For this review, take the finished solid that the model builds, in its own axes (mm). Coordinates: 2 decimals unless noted, no trailing zeros. Loops run counter-clockwise (first coordinate to the right, second up) from the corner with the lowest first, then second, coordinate; pieces in that order, holes last. Notation, with made-up numbers: (57.5, -33.5) -> (88.5, -33.5) arc R28 cw to (88.5, -5.5) -> close; hole circle Ø10 at (24, -35.5). An arc over 180 degrees is marked (long way). Use a Markdown table: item, result.
Autodesk Inventor part; units mm, degrees
ref_plane "YZ Plane" through (0, 0, 0) normal (1, 0, 0) x (0, 1, 0)
ref_plane "XZ Plane" through (0, 0, 0) normal (0, 1, 0) x (-1, 0, 0)
ref_plane "XY Plane" through (0, 0, 0) normal (0, 0, 1) x (1, 0, 0)
sketch "Sketch1" plane through (0, 0, 0) normal (0, 1, 0) x (-1, 0, 0)
  line L0 (0, 0) -> (50, 0)
  line L1 (50, 0) -> (50, -58)
  line L2 (50, -58) -> (0, -58)
  line L3 (0, -58) -> (0, 0)
  line L4 (46, 11.182) -> (46, -76.3332) construction
  line L5 (62.4819, -54) -> (-10.7264, -54) construction
  point P0 (46, -18)
  point P1 (18, -54)
  dimension "d0" = 50
  dimension "d1" = 58
  dimension "d2" = 4
  dimension "d3" = 4
  dimension "d4" = 18
  dimension "d5" = 18
extrude "Extrusion1" add sketch "Sketch1" against normal blind 3
hole "Hole1" at (-46, 0, -18) at (-18, 0, -54) direction (0, -1, 0) diameter 3.2 end through all
properties part number "Step-back cover -electronics enc"
(1) Take a section at B-B on z = -54. Write out the cut boundary in (x, y), plus the area to 3 significant figures.
Found:
| item | result |
|---|---|
| outline | (-50, -3) -> (-19.6, -3) -> (-19.6, 0) -> (-50, 0) -> close; (-16.4, -3) -> (0, -3) -> (0, 0) -> (-16.4, 0) -> close |
| area | 140 mm^2 |
(2) For line 1 along Z through (x, y) = (-46, -1.7); line 2 along X through (y, z) = (-1.5, -18); line 3 along Z through (x, y) = (-18, -2.35), list the stretches that pass through material, from the lowest coordinate up.
Found:
| item | result |
|---|---|
| line 1 | z = -58 to -19.6, -16.4 to 0 |
| line 2 | x = -50 to -47.6, -44.4 to 0 |
| line 3 | z = -58 to -55.6, -52.4 to 0 |
(3) Take a section at A-A on x = -18. Write out the cut boundary in (y, z), plus the area to 3 significant figures.
Found:
| item | result |
|---|---|
| outline | (-3, -58) -> (0, -58) -> (0, -55.6) -> (-3, -55.6) -> close; (-3, -52.4) -> (0, -52.4) -> (0, 0) -> (-3, 0) -> close |
| area | 164 mm^2 |
(4) Mouldability with a two-part tool opening along X and no side actions: class faces 1 (the face through (-19.35, -1.52, -53.14)), 2 (the face through (0, -1, -29)), 3 (the face through (-25, 0, -29)), 4 (the face through (-50, -1, -29)) as pulls with the +X half, pulls with the -X half, needs draft (parallel to the pull), parting line crosses it, or undercut.
Found:
| item | result |
|---|---|
| face 1 | undercut |
| face 2 | pulls with the +X half |
| face 3 | needs draft |
| face 4 | pulls with the -X half |
